Verification items for the finished model (mm, model axes). Face numbers are marked on the shaded views. A direction names the side the tool comes from. Give positions to 0.01 mm unless a question says otherwise; leave off trailing zeros. Loops run counter-clockwise (first coordinate to the right, second up) from the corner with the lowest first, then second, coordinate; pieces in that order, holes last. Notation, with made-up numbers: (86, 55) - (124, 55) arc R20 cw to (124, 87) - close; hole circle Ø11 at (-36.5, 76.25). An arc over 180 degrees is marked (long way). One line per item, written item: value. Start each with the question number.
1. Mould release check, pull along Y, two halves, no side actions. Record for the marked faces 4, 5 and 6: pulls with the +Y half, pulls with the -Y half, needs draft (parallel to the pull), parting line crosses it, or undercut.
2. Sectioned sample at D-D (x = -4). Record the cut outline in (y, z).
3. Gauge pin test, flat ends, axial feed: pin 1 (1.4 mm diameter, centred on y = 0, z = -4.5, fed in from -X); pin 2 (1.5 mm diameter, centred on y = 0, z = -3, fed in from +X). Record the tip position at first contact, or that the pin passes through.
4. Sectioned sample at A-A (z = 0.5). Record the cut outline in (x, y), plus the area to 3 significant figures.
5. Scan lines: L1, parallel to X at y = 1.5, z = 2.75; L2, parallel to Z at x = -3.65, y = 0; L3, parallel to X at y = 0, z = -2.25 (3 decimals). Record each from-to range of solid material in increasing order. Write a range as [from, to].
6. Access from +Z, -Z, +X, -X, +Y, -Y to the whole of each face (thin tool, end or side, straight path). Record for the marked faces 1, 2 and 3.
7. Sectioned sample at B-B (y = 0). Record the cut outline in (x, z) (3 decimals), plus the area to 3 significant figures.
8. Sectioned sample at C-C (x = 0). Record the cut outline in (y, z) (3 decimals), plus the area to 4 significant figures.
from build123d import *

# Parameters (mm, degrees)
PAD_DEPTH    = 4
PAD001_DEPTH = 2
SKETCH002_R  = 5
PAD002_DEPTH = 7
SKETCH003_R  = 1.15
POCKET_DEPTH = 5


with BuildPart() as part:
    # Sketch → Pad (new body)
    with BuildSketch(Plane.XY):
        with BuildLine():
            Line((-4.25, 8), (4.25, 8))
            ThreePointArc((8, 4.25), (6.90165, 6.90165), (4.25, 8))
            Line((8, 4.25), (8, -4.25))
            ThreePointArc((4.25, -8), (6.90165, -6.90165), (8, -4.25))
            Line((4.25, -8), (-4.25, -8))
            ThreePointArc((-8, -4.25), (-6.90165, -6.90165), (-4.25, -8))
            Line((-8, -4.25), (-8, 4.25))
            ThreePointArc((-4.25, 8), (-6.90165, 6.90165), (-8, 4.25))
        make_face()
        with BuildLine():
            Line((-4.5, 6), (4.5, 6))
            ThreePointArc((6, 4.5), (5.56066, 5.56066), (4.5, 6))
            Line((6, 4.5), (6, -4.5))
            ThreePointArc((4.5, -6), (5.56066, -5.56066), (6, -4.5))
            Line((4.5, -6), (-4.5, -6))
            ThreePointArc((-6, -4.5), (-5.56066, -5.56066), (-4.5, -6))
            Line((-6, -4.5), (-6, 4.5))
            ThreePointArc((-4.5, 6), (-5.56066, 5.56066), (-6, 4.5))
        make_face(mode=Mode.SUBTRACT)
    extrude(amount=PAD_DEPTH)

    # Sketch001 → Pad001 (join)
    with BuildSketch(Plane.XY):
        with BuildLine():
            Line((-4.25, 8), (4.25, 8))
            ThreePointArc((8, 4.25), (6.90165, 6.90165), (4.25, 8))
            Line((8, 4.25), (8, -4.25))
            ThreePointArc((4.25, -8), (6.90165, -6.90165), (8, -4.25))
            Line((4.25, -8), (-4.25, -8))
            ThreePointArc((-8, -4.25), (-6.90165, -6.90165), (-4.25, -8))
            Line((-8, -4.25), (-8, 4.25))
            ThreePointArc((-4.25, 8), (-6.90165, 6.90165), (-8, 4.25))
        make_face()
        with BuildLine():
            ThreePointArc((-2.15, -1.50603), (2.625, 0), (-2.15, 1.50603))
            Line((-2.15, 1.50603), (-2.15, -1.50603))
        make_face(mode=Mode.SUBTRACT)
    extrude(amount=-PAD001_DEPTH)

    # Sketch002 → Pad002 (join)
    with BuildSketch(Plane(origin=(0, 0, 0), x_dir=(-1, 0, 0), z_dir=(0, 0, 1))):
        Circle(SKETCH002_R)
        with BuildLine():
            ThreePointArc((2.15, 1.50603), (-2.625, 0), (2.15, -1.50603))
            Line((2.15, 1.50603), (2.15, -1.50603))
        make_face(mode=Mode.SUBTRACT)
    extrude(amount=-PAD002_DEPTH)

    # Sketch003 → Pocket (cut)
    with BuildSketch(Plane(origin=(0, 0, -4.5), x_dir=(0, 1, 0), z_dir=(1, 0, 0))):
        Circle(SKETCH003_R)
    extrude(amount=-POCKET_DEPTH, mode=Mode.SUBTRACT)


solid = part.part
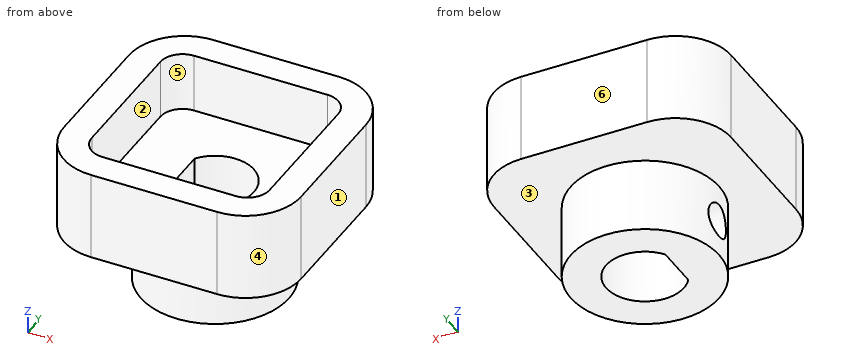
Results are:
1. face 4: pulls with the -Y half
1. face 5: undercut
1. face 6: pulls with the +Y half
2. outline: (-8, -2) - (-3, -2) - (-3, -7) - (3, -7) - (3, -2) - (8, -2) - (8, 4) - (6, 4) - (6, 0) - (-6, 0) - (-6, 4) - (-8, 4) - close; hole circle Ø2.3 at (0, -4.5)
3. pin 1: stops at x = 2.53
3. pin 2: stops at x = 5
4. outline: (-8, -4.25) arc R3.75 ccw to (-4.25, -8) - (4.25, -8) arc R3.75 ccw to (8, -4.25) - (8, 4.25) arc R3.75 ccw to (4.25, 8) - (-4.25, 8) arc R3.75 ccw to (-8, 4.25) - close; hole (-6, -4.5) arc R1.5 ccw to (-4.5, -6) - (4.5, -6) arc R1.5 ccw to (6, -4.5) - (6, 4.5) arc R1.5 ccw to (4.5, 6) - (-4.5, 6) arc R1.5 ccw to (-6, 4.5) - close
4. area: 102 mm^2
5. L1: x = [-8, -6], [6, 8]
5. L2: z = [-7, -5.65], [-3.35, 0]
5. L3: x = [-5, -2.15], [2.625, 5]
6. face 1: +Z, -Z, +X, +Y, -Y
6. face 2: +Z
6. face 3: -Z
7. outline: (-8, -2) - (-5, -2) - (-5, -3.35) - (-2.15, -3.35) - (-2.15, 0) - (-6, 0) - (-6, 4) - (-8, 4) - close; (-5, -7) - (-2.15, -7) - (-2.15, -5.65) - (-5, -5.65) - close; (2.625, -7) - (5, -7) - (5, -2) - (8, -2) - (8, 4) - (6, 4) - (6, 0) - (2.625, 0) - close
7. area: 58.0 mm^2
8. outline: (-8, -2) - (-5, -2) - (-5, -7) - (-2.625, -7) - (-2.625, 0) - (-6, 0) - (-6, 4) - (-8, 4) - close; (2.625, -7) - (5, -7) - (5, -2) - (8, -2) - (8, 4) - (6, 4) - (6, 0) - (2.625, 0) - close
8. area: 61.25 mm^2
